Can you work these out from the drawing? Everything is in mm from the part's minimum corner. A direction names the side the tool comes from. Round coordinates to 2 decimals unless told otherwise and drop trailing zeros. Loops run counter-clockwise (first coordinate to the right, second up) from the corner with the lowest first, then second, coordinate; pieces in that order, holes last. Notation, with made-up numbers: (26.5, 74) - (33.5, 74) arc R30 ccw to (33.5, 109) - close; hole circle Ø1 at (28, -0.75). An arc over 180 degrees is marked (long way). Return JSON: item names as keys, results as strings. Group by question number.
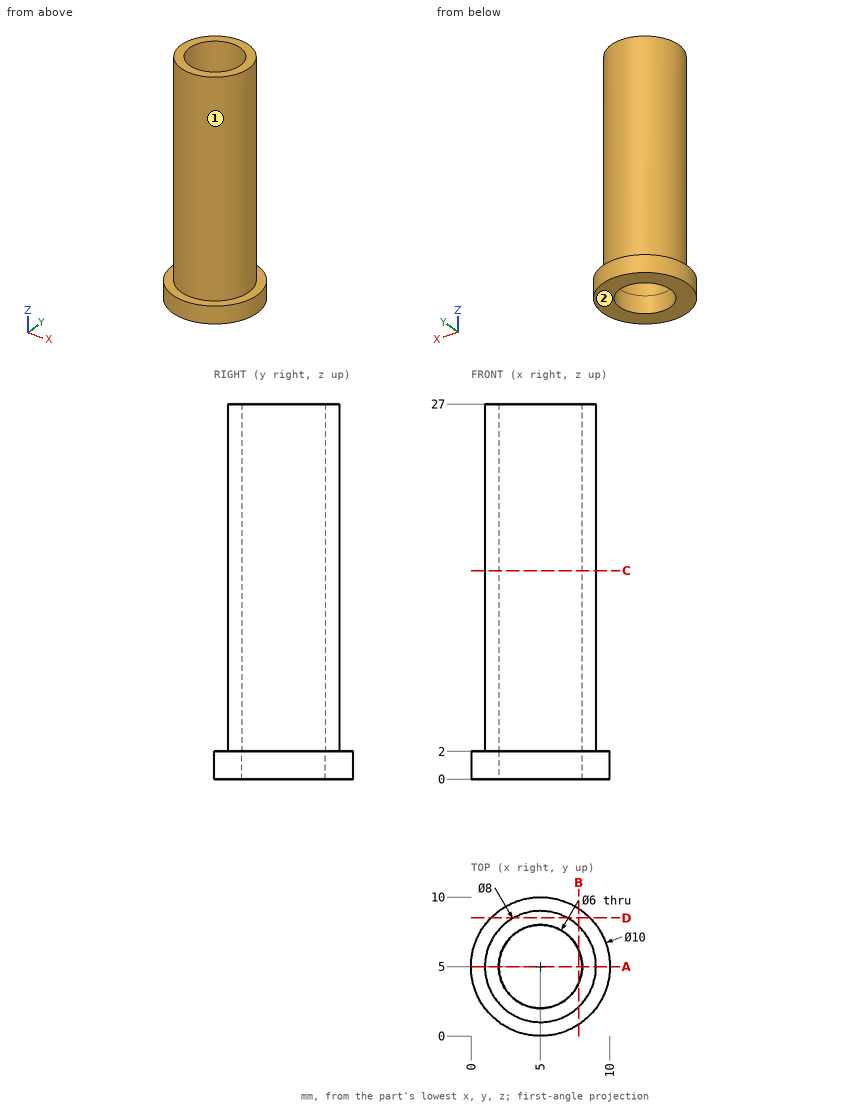
Q1. Imagine slicing it at C-C, the plane z = 15. List the corners of the cut face in (x, y) for me, and give its area (3 significant figures).
Q2. Imagine slicing it at D-D, the plane y = 8.5. List the corners of the cut face in (x, z) for me.
Q3. For the marked faces 1 and 2, which set-ups out of +Z, -Z, +X, -X, +Y, -Y let a thin tool reach every point of the face, with its end or its side?
Q4. Will these pins go through, and if not, where does the flat tip stop? pin 1 Ø5 at (x, y) = (4, 8) entering from -Z; pin 2 Ø1 at (y, z) = (7, 10.5) entering from +X; pin 3 Ø3 at (y, z) = (2.5, 15) entering from -X; pin 4 Ø6 at (y, z) = (3.5, 7.5) entering from -X.
Q5. Imagine slicing it at B-B, the plane x = 7.75. List the corners of the cut face in (y, z) for me.
Q6. Please list where these lines run through material, in increasing order: line 1 (Y direction, x = 5, z = 17.25); line 2 (Y direction, x = 5, z = 1); line 3 (X direction, y = 5.5, z = 14.75).
Q7. Imagine slicing it at A-A, the plane y = 5. List the corners of the cut face in (x, z) for me, and give its area (3 significant figures).
Output values:
{
 "1": {"outline": "circle Ø8 at (5, 5); hole circle Ø6 at (5, 5)", "area": "22.0 mm^2"},
 "2": {"outline": "(1.43, 0) - (8.57, 0) - (8.57, 2) - (6.94, 2) - (6.94, 27) - (3.06, 27) - (3.06, 2) - (1.43, 2) - close"},
 "3": {"face 1": "+Z", "face 2": "-Z, +X, -X, +Y, -Y"},
 "4": {"pin 1": "stops at z = 0", "pin 2": "stops at x = 8.71", "pin 3": "stops at x = 1.13", "pin 4": "stops at x = 1"},
 "5": {"outline": "(0.82, 0) - (3.8, 0) - (3.8, 27) - (2.1, 27) - (2.1, 2) - (0.82, 2) - close; (6.2, 0) - (9.18, 0) - (9.18, 2) - (7.9, 2) - (7.9, 27) - (6.2, 27) - close"},
 "6": {"line 1": "y = 1 to 2, 8 to 9", "line 2": "y = 0 to 2, 8 to 10", "line 3": "x = 1.03 to 2.04, 7.96 to 8.97"},
 "7": {"outline": "(0, 0) - (2, 0) - (2, 27) - (1, 27) - (1, 2) - (0, 2) - close; (8, 0) - (10, 0) - (10, 2) - (9, 2) - (9, 27) - (8, 27) - close", "area": "58.0 mm^2"}
}
